Could you check a few things on this model? Use its own coordinates, in mm. A direction names the side the tool comes from. Give positions to 0.01 mm unless a question says otherwise; leave off trailing zeros. Write each loop counter-clockwise with the first axis right and the second up, starting at its lowest first coordinate (ties: lowest second). Pieces come first, ordered by that corner, then holes. Notation, with made-up numbers: (21.5, -14.5) - (55.5, -14.5) arc R17 ccw to (55.5, -6.5) - close; hole circle Ø5 at (-33.75, -2.75). An arc over 180 degrees is marked (long way). Write item = value, one per line.
from build123d import *

# Parameters (mm, degrees)
AXLE_BASE_SKETCH_R        = 25.5
AXLE_DEPTH                = 68.5
GUARD_BASE_R              = 37.5
GUARD_DEPTH               = 5
INNER_AXLE_HOLE_BASE_R    = 10
INNER_AXLE_HOLE_DEPTH     = 74.5
BEND_START                = -55.75
BEND_ROOM_BASE_W          = 1.5
BEND_ROOM_BASE_H          = 75
BEND_ROOM_1_DEPTH         = 55.750001
BEND_ROOM_2_COUNT         = 2
BEND_ROOM_2_ANGLE         = 90
EASY_REMOVAL_CHAMFER_SIZE = 4


with BuildPart() as part:
    # Axle base sketch → Axle (new body)
    with BuildSketch(Plane.XY):
        Circle(AXLE_BASE_SKETCH_R)
    extrude(amount=AXLE_DEPTH)

    # Guard base → Guard (add)
    with BuildSketch(Plane(origin=(0, 0, 0), x_dir=(-1, 0, 0), z_dir=(0, 0, -1))):
        Circle(GUARD_BASE_R)
    extrude(amount=GUARD_DEPTH)

    # Inner axle hole base → Inner axle hole (cut, through all)
    with BuildSketch(Plane.XY.offset(68.5)):
        Circle(INNER_AXLE_HOLE_BASE_R)
    extrude(amount=-INNER_AXLE_HOLE_DEPTH, mode=Mode.SUBTRACT)

    # Mate ring base → Mate rings (revolve)
    with BuildSketch(Plane(origin=(0, 0, 0), x_dir=(1, 0, 0), z_dir=(0, 1, 0))):
        Polygon((25.5, -68.5), (26.25, -67.75), (26.25, -67), (25.5, -66.25), align=None)
        Polygon((25.5, -62.75), (26.25, -62), (26.25, -61.25), (25.5, -60.5), align=None)
    revolve(axis=Axis((0, 0, 0), (0, 0, -1)))

    # Inner mass remove base → Inner mass remove (revolve, cut)
    with BuildSketch(Plane(origin=(0, 0, 0), x_dir=(0, 0, -1), z_dir=(1, 0, 0))):
        Polygon((-68.5, 0), (-50.75, -17.75), (-12.75, -17.75), (5, 0), align=None)
    revolve(axis=Axis((0, 0, 0), (0, 0, -1)), mode=Mode.SUBTRACT)

    # Bend room base → Bend room 1 (cut)
    with BuildSketch(Plane.XY.offset(68.5).offset(BEND_START)):
        Rectangle(BEND_ROOM_BASE_W, BEND_ROOM_BASE_H)
    bend_room_1 = extrude(amount=BEND_ROOM_1_DEPTH, mode=Mode.SUBTRACT)

    # Bend room 2: Bend room 1 ×2 about axis
    bend_room_2_axis = Axis((0, 0, 0), (0, 0, -1))
    for i in range(1, BEND_ROOM_2_COUNT):
        add(bend_room_1.rotate(bend_room_2_axis, i * BEND_ROOM_2_ANGLE / (BEND_ROOM_2_COUNT - 1)), mode=Mode.SUBTRACT)

    # Easy removal chamfer
    easy_removal_chamfer_edges = [part.edges().sort_by_distance(p)[0] for p in [
        (37.5, 0, 0),
    ]]
    chamfer(easy_removal_chamfer_edges, length=EASY_REMOVAL_CHAMFER_SIZE)


solid = part.part
1. Thinking about a two-plate mould opening in X: for faces 1 (the face through (-9.14, -9.34, 55.43)), 2 (the face through (-0.75, 20, 46)), 3 (the face through (18.22, 17.84, 64.48)), 4 (the face through (-17.92, -18.31, 60.62)), which applies, pulls with the +X half, pulls with the -X half, needs draft (parallel to the pull), parting line crosses it, or undercut?
Filled sheet:
face_1 = undercut
face_2 = undercut
face_3 = pulls with the +X half
face_4 = pulls with the -X half
2. If we section it at A-A, the plane z = 43.5: Please give me the cut outline in (x, y).
Filled sheet:
outline = (-25.49, -0.75) arc R25.5 ccw to (-0.75, -25.49) - (-0.75, -17.73) arc R17.75 cw to (-17.73, -0.75) - close; (-25.49, 0.75) - (-17.73, 0.75) arc R17.75 cw to (-0.75, 17.73) - (-0.75, 25.49) arc R25.5 ccw to start; (0.75, -25.49) arc R25.5 ccw to (25.49, -0.75) - (17.73, -0.75) arc R17.75 cw to (0.75, -17.73) - close; (0.75, 17.73) arc R17.75 cw to (17.73, 0.75) - (25.49, 0.75) arc R25.5 ccw to (0.75, 25.49) - close
3. I need wall thicknesses on line 1 (Y direction, x = 0, z = 2); line 2 (Z direction, x = -18.5, y = -26); line 3 (X direction, y = -16.5, z = 31.5). Which ranges of each line are inside material? Lowest first, please.
Filled sheet:
line_1 = -25.5 to -10, 10 to 25.5
line_2 = -5 to 0
line_3 = -19.44 to -6.54, 6.54 to 19.44
4. For pin 1 (13 mm diameter, centred on x = 16, z = 51, fed in from +Y); pin 2 (5 mm diameter, centred on x = -6.5, y = 6.5, fed in from +Z); pin 3 (8 mm diameter, centred on y = 14, z = 54, fed in from -X); pin 4 (0.5 mm diameter, centred on x = -20, y = 0, fed in from +Z), each with a flat end and sliding along its axis, tell me the tip position at first contact or that it passes through.
Filled sheet:
pin_1 = 23.66
pin_2 = 68.5
pin_3 = -23.46
pin_4 = 12.75
5. Which directions (+Z, -Z, +X, -X, +Y, -Y) give clear straight access to the entire face, cutting with the end or side of a thin tool? Please do faces 5 (the face through (0.75, -20, 46)), 6 (the face through (-18.76, 18.36, 67.37)), 7 (the face through (-5.5, -24.9, 29.8)).
Filled sheet:
face_5 = +Z, +Y, -Y
face_6 = +Z, -X, +Y
face_7 = none
